from build123d import *

# Parameters (mm, degrees)
ESTRUSIONE_ESTRUSIONE1_DEPTH = 8
SCHIZZO2_W                   = 14
SCHIZZO2_H                   = 5.5
ESTRUSIONE_ESTRUSIONE2_DEPTH = 9.208407085
SCHIZZO3_W                   = 6
SCHIZZO3_H                   = 5.5
ESTRUSIONE_ESTRUSIONE3_DEPTH = 5.291592915
SCHIZZO4_W                   = 14
SCHIZZO4_H                   = 14.5
ESTRUSIONE_ESTRUSIONE4_DEPTH = 5.5
ESTRUSIONE_ESTRUSIONE5_DEPTH = 4.5
TAGLIO_ESTRUSIONE1_DEPTH     = 8
TAGLIO_ESTRUSIONE2_DEPTH     = 5.5
SCHIZZO8_W                   = 14
SCHIZZO8_H                   = 19
ESTRUSIONE_ESTRUSIONE6_DEPTH = 23.5
ESTRUSIONE_ESTRUSIONE7_DEPTH = 10.5
TAGLIO_ESTRUSIONE3_DEPTH     = 4.5
TAGLIO_ESTRUSIONE4_DEPTH     = 1
TAGLIO_ESTRUSIONE5_DEPTH     = 4.5
SCHIZZO13_W                  = 23.5
SCHIZZO13_H                  = 25
ESTRUSIONE_ESTRUSIONE8_DEPTH = 6
SCHIZZO14_W                  = 6
SCHIZZO14_H                  = 1
TAGLIO_ESTRUSIONE6_DEPTH     = 5
TAGLIO_ESTRUSIONE7_DEPTH     = 14
SCHIZZO16_W                  = 6
SCHIZZO16_H                  = 1
TAGLIO_ESTRUSIONE8_DEPTH     = 5
RACCORDO1_R                  = 2


with BuildPart() as part:
    # Schizzo1 → Estrusione-Estrusione1 (new body)
    with BuildSketch(Plane(origin=(4, 0, 0), x_dir=(0, 0, -1), z_dir=(1, 0, 0))):
        Polygon((-5.5, -9.5), (-5.5, -4.208407085), (-11, -4.208407085), align=None)
    extrude(amount=-ESTRUSIONE_ESTRUSIONE1_DEPTH)

    # Schizzo2 → Estrusione-Estrusione2 (add)
    with BuildSketch(Plane(origin=(0, -4.208407085, 0), x_dir=(-1, 0, 0), z_dir=(0, 1, 0))):
        with Locations((3, 8.25)):
            Rectangle(SCHIZZO2_W, SCHIZZO2_H)
    extrude(amount=ESTRUSIONE_ESTRUSIONE2_DEPTH)

    # Schizzo3 → Estrusione-Estrusione3 (add)
    with BuildSketch(Plane.XZ.offset(4.208407085)):
        with Locations((-7, 8.25)):
            Rectangle(SCHIZZO3_W, SCHIZZO3_H)
    extrude(amount=ESTRUSIONE_ESTRUSIONE3_DEPTH)

    # Schizzo4 → Estrusione-Estrusione4 (add)
    with BuildSketch(Plane(origin=(0, 0, 5.5), x_dir=(-1, 0, 0), z_dir=(0, 9.448610433574674e-12, -1.0))):
        with Locations((3, -2.25)):
            Rectangle(SCHIZZO4_W, SCHIZZO4_H)
    extrude(amount=ESTRUSIONE_ESTRUSIONE4_DEPTH)

    # Schizzo5 → Estrusione-Estrusione5 (add)
    with BuildSketch(Plane(origin=(0, 5, 0), x_dir=(-1, 0, 0), z_dir=(0, 1, 0))):
        with BuildLine():
            Line((10, 0), (-4, 0))
            add(Edge.make_bspline(
                [(-4, 4.5), (-4, 3), (-4, 1.5), (-4, 0)],
                knots=[0, 0, 0, 0, 1, 1, 1, 1], degree=3))
            Line((-4, 4.5), (-4, 11))
            Line((-4, 11), (10, 11))
            add(Edge.make_bspline(
                [(10, 11), (10, 9.166666667), (10, 7.333333333), (10, 5.5)],
                knots=[0, 0, 0, 0, 1, 1, 1, 1], degree=3))
            add(Edge.make_bspline(
                [(10, 5.5), (10, 5.166666667), (10, 4.833333333), (10, 4.5)],
                knots=[0, 0, 0, 0, 1, 1, 1, 1], degree=3))
            add(Edge.make_bspline(
                [(10, 4.5), (10, 3), (10, 1.5), (10, 0)],
                knots=[0, 0, 0, 0, 1, 1, 1, 1], degree=3))
        make_face()
    extrude(amount=ESTRUSIONE_ESTRUSIONE5_DEPTH)

    # Schizzo6 → Taglio-Estrusione1 (cut)
    with BuildSketch(Plane(origin=(4, 0, 0), x_dir=(0, 0, -1), z_dir=(1, 0, 0))):
        Polygon((-11, 4.208407085), (-5.5, 9.5), (-11, 9.5), align=None)
    extrude(amount=-TAGLIO_ESTRUSIONE1_DEPTH, mode=Mode.SUBTRACT)

    # Schizzo7 → Taglio-Estrusione2 (cut)
    with BuildSketch(Plane.XY.offset(11)):
        with BuildLine():
            Line((-10, -9.5), (-4, -9.5))
            Line((-4, -9.5), (-4, 9.5))
            Line((-4, 9.5), (-10, 9.5))
            add(Edge.make_bspline(
                [(-10, 9.5), (-10, 8), (-10, 6.5), (-10, 5)],
                knots=[0, 0, 0, 0, 1, 1, 1, 1], degree=3))
            Line((-10, 5), (-10, -9.5))
        make_face()
    extrude(amount=-TAGLIO_ESTRUSIONE2_DEPTH, mode=Mode.SUBTRACT)

    # Schizzo8 → Estrusione-Estrusione6 (add)
    with BuildSketch(Plane(origin=(0, 0, 0), x_dir=(-1, 0, 0), z_dir=(0, 3.448151725834727e-12, -1.0))):
        with Locations((3, 0)):
            Rectangle(SCHIZZO8_W, SCHIZZO8_H)
    extrude(amount=ESTRUSIONE_ESTRUSIONE6_DEPTH)

    # Schizzo9 → Estrusione-Estrusione7 (add)
    with BuildSketch(Plane.XZ.offset(9.5)):
        with BuildLine():
            Line((4, -23.5), (-10, -23.5))
            Line((-10, -23.5), (-10, 0))
            add(Edge.make_bspline(
                [(-10, 4.5), (-10, 3), (-10, 1.5), (-10, 0)],
                knots=[0, 0, 0, 0, 1, 1, 1, 1], degree=3))
            add(Edge.make_bspline(
                [(-10, 5.5), (-10, 5.166666667), (-10, 4.833333333), (-10, 4.5)],
                knots=[0, 0, 0, 0, 1, 1, 1, 1], degree=3))
            Line((-10, 5.5), (4, 5.5))
            add(Edge.make_bspline(
                [(4, 5.5), (4, 5.166666667), (4, 4.833333333), (4, 4.5)],
                knots=[0, 0, 0, 0, 1, 1, 1, 1], degree=3))
            add(Edge.make_bspline(
                [(4, 4.5), (4, 3), (4, 1.5), (4, 0)],
                knots=[0, 0, 0, 0, 1, 1, 1, 1], degree=3))
            Line((4, 0), (4, -23.5))
        make_face()
    extrude(amount=ESTRUSIONE_ESTRUSIONE7_DEPTH)

    # Schizzo10 → Taglio-Estrusione3 (cut)
    with BuildSketch(Plane(origin=(0, 9.5, 0), x_dir=(-1, 0, 0), z_dir=(0, 1, 0))):
        with BuildLine():
            Line((10, -23.5), (10, 0))
            add(Edge.make_bspline(
                [(10, 4.5), (10, 3), (10, 1.5), (10, 0)],
                knots=[0, 0, 0, 0, 1, 1, 1, 1], degree=3))
            add(Edge.make_bspline(
                [(10, 5.5), (10, 5.166666667), (10, 4.833333333), (10, 4.5)],
                knots=[0, 0, 0, 0, 1, 1, 1, 1], degree=3))
            Line((10, 5.5), (4, 5.5))
            Line((4, 5.5), (4, 4.5))
            Line((4, 4.5), (-4, 4.5))
            add(Edge.make_bspline(
                [(-4, 4.5), (-4, 3), (-4, 1.5), (-4, 0)],
                knots=[0, 0, 0, 0, 1, 1, 1, 1], degree=3))
            Line((-4, 0), (-4, -23.5))
            Line((-4, -23.5), (10, -23.5))
        make_face()
    extrude(amount=-TAGLIO_ESTRUSIONE3_DEPTH, mode=Mode.SUBTRACT)

    # Schizzo11 → Taglio-Estrusione4 (cut)
    with BuildSketch(Plane.XY.offset(5.5)):
        Polygon((-4, -9.5), (-4, 5), (-10, 5), (-10, -20), (4, -20), (4, -9.5), align=None)
    extrude(amount=-TAGLIO_ESTRUSIONE4_DEPTH, mode=Mode.SUBTRACT)

    # Schizzo12 → Taglio-Estrusione5 (cut)
    with BuildSketch(Plane.XY.offset(4.5)):
        Polygon((4, 4), (4, 5), (-10, 5), (-10, -20), (4, -20), (4, -4), (-4, -4), (-4, 4), align=None)
    extrude(amount=-TAGLIO_ESTRUSIONE5_DEPTH, mode=Mode.SUBTRACT)

    # Schizzo13 → Estrusione-Estrusione8 (add)
    with BuildSketch(Plane(origin=(4, 0, 0), x_dir=(0, 0, -1), z_dir=(1, 0, 0))):
        with Locations((11.75, -7.5)):
            Rectangle(SCHIZZO13_W, SCHIZZO13_H)
    extrude(amount=ESTRUSIONE_ESTRUSIONE8_DEPTH)

    # Schizzo14 → Taglio-Estrusione6 (cut)
    with BuildSketch(Plane.ZY.offset(10)):
        with Locations((-16.5, -15.5)):
            Rectangle(SCHIZZO14_W, SCHIZZO14_H)
    extrude(amount=-TAGLIO_ESTRUSIONE6_DEPTH, mode=Mode.SUBTRACT)

    # Schizzo15 → Taglio-Estrusione7 (cut)
    with BuildSketch(Plane.XZ.offset(20)):
        with BuildLine():
            Line((3.1, -11.9000249), (3.1, -8.0999751))
            ThreePointArc((3.1, -8.0999751), (0, -4.9999751), (-3.1, -8.0999751))
            Line((-3.1, -8.0999751), (-3.1, -11.9000249))
            ThreePointArc((-3.1, -11.9000249), (0, -15.0000249), (3.1, -11.9000249))
        make_face()
    extrude(amount=-TAGLIO_ESTRUSIONE7_DEPTH, mode=Mode.SUBTRACT)

    # Schizzo16 → Taglio-Estrusione8 (cut)
    with BuildSketch(Plane(origin=(10, 0, 0), x_dir=(0, 0, -1), z_dir=(1, 0, 0))):
        with Locations((16.5, -15.5)):
            Rectangle(SCHIZZO16_W, SCHIZZO16_H)
    extrude(amount=-TAGLIO_ESTRUSIONE8_DEPTH, mode=Mode.SUBTRACT)

    # Raccordo1
    raccordo1_edges = [part.edges().sort_by_distance(p)[0] for p in [
        (-10, -2.25, -23.5),
        (10, -7.5, -23.5),
    ]]
    fillet(raccordo1_edges, radius=RACCORDO1_R)


solid = part.part
Work out the finished part from the listing and answer in its coordinate system (mm). A direction names the side the tool comes from. Give positions to 0.01 mm unless a question says otherwise; leave off trailing zeros. Loops run counter-clockwise (first coordinate to the right, second up) from the corner with the lowest first, then second, coordinate; pieces in that order, holes last. Notation, with made-up numbers: (-8, 86) -> (25, 86) arc R23 cw to (25, 120) -> close; hole circle Ø9 at (73, 35). An arc over 180 degrees is marked (long way). Use a Markdown table: item, result. Add a question column.
1. Section C-C on z = -3 is taken. Determine the outline of the cut face in (x, y).
2. Section D-D on z = 2 is taken. Determine the outline of the cut face in (x, y), and give its area (3 significant figures).
3. Find the intervals of material crossed by probe 1 along Y at (x, z) = (7, -17); probe 2 along Z at (x, y) = (6, -15.5); probe 3 along Z at (x, y) = (-6.5, 3.5), in increasing order.
4. Section A-A on y = -9 is taken. Determine the outline of the cut face in (x, z), and give its area (3 significant figures).
5. Section B-B on x = 0 is taken. Determine the outline of the cut face in (y, z).
6. Determine the mould class of faces 1 (the flat face through (-3.1, -13, -10)), 2 (the flat face through (-8, -16, -17)), 3 (the flat face through (5, -15.5, -16.5)) for opening direction X: released by +X, released by -X, zero draft, split by the parting line, or undercut.
7. Flat-ended cylindrical pins translate along their axes: pin 1 Ø3 at (x, z) = (1, -6) entering from +Y; pin 2 Ø2 at (x, z) = (-0.5, 3) entering from -Y; pin 3 Ø0.5 at (x, y) = (-8.5, -15.5) entering from +Z. Find the tip coordinate at first contact, or state that the pin passes through.
8. For faces 4 (the flat face through (-7.5, -15.5, -19.5)), 5 (the cylindrical face through (0, -13, -5)), 6 (the flat face through (0, 4, 2)), 7 (the flat face through (7.5, -15.5, -13.5)), determine the directions among +Z, -Z, +X, -X, +Y, -Y from which every point of the face is accessible in a straight line to the end or side of a thin tool.
Results below:
| question | item | result |
|---|---|---|
| 1 | outline | (-10, -20) -> (10, -20) -> (10, 5) -> (-10, 5) -> close |
| 2 | outline | (-4, -4) -> (4, -4) -> (4, 4) -> (-4, 4) -> close |
| 2 | area | 64.0 mm^2 |
| 3 | probe 1 | y = -20 to -16, -15 to 5 |
| 3 | probe 2 | z = -23.5 to -19.5, -13.5 to 0 |
| 3 | probe 3 | z = -23.5 to 0 |
| 4 | outline | (-10, -21.5) arc R2 ccw to (-8, -23.5) -> (8, -23.5) arc R2 ccw to (10, -21.5) -> (10, 0) -> (-10, 0) -> close; (-4, 4.5) -> (4, 4.5) -> (4, 6.02) -> (-4, 6.02) -> close; hole (-3.1, -11.9) arc R3.1 ccw to (3.1, -11.9) -> (3.1, -8.1) arc R3.1 ccw to (-3.1, -8.1) -> close |
| 4 | area | 427 mm^2 |
| 5 | outline | (-20, -23.5) -> (5, -23.5) -> (5, 0) -> (4, 0) -> (4, 4.5) -> (9.5, 4.5) -> (9.5, 5.5) -> (4.21, 11) -> (-4.21, 11) -> (-9.5, 5.5) -> (-9.5, 4.5) -> (-4, 4.5) -> (-4, 0) -> (-20, 0) -> (-20, -5) -> (-6, -5) -> (-6, -15) -> (-20, -15) -> close |
| 6 | face 1 | undercut |
| 6 | face 2 | zero draft |
| 6 | face 3 | released by +X |
| 7 | pin 1 | stops at y = 5 |
| 7 | pin 2 | stops at y = -4 |
| 7 | pin 3 | stops at z = 0 |
| 8 | face 4 | -X |
| 8 | face 5 | -Y |
| 8 | face 6 | +X, -X, +Y |
| 8 | face 7 | +X |
